Geometry: final body of the model. Coordinates: model frame, mm. Coordinates: 2 decimals unless noted, no trailing zeros. Write each loop counter-clockwise with the first axis right and the second up, starting at its lowest first coordinate (ties: lowest second). Pieces come first, ordered by that corner, then holes. Notation, with made-up numbers: (-22.75, 15) - (-13.75, 15) arc R9 cw to (-13.75, 22) - close; hole circle Ø2 at (36, 38). An arc over 180 degrees is marked (long way). Answer as a JSON object with one key per item and string values. Group by question number.
Item 1: Section A-A on y = 3.15. Return loops of the section in (x, z).
Item 2: First-contact query: pin 1 Ø2.5 at (x, y) = (-7.5, 3.5) entering from +Z; pin 2 Ø3 at (y, z) = (3.5, 14) entering from +X; pin 3 Ø1.5 at (y, z) = (3, -24.5) entering from +X. Flat tips, straight axial feed; report the tip coordinate or a pass-through.
Item 3: Section B-B on x = -16. Return loops of the section in (y, z), and give its area (4 significant figures).
Item 4: Line query: line 1 along Z through (x, y) = (5, 4.55); line 2 along X through (y, z) = (4.05, 21.5); line 3 along X through (y, z) = (3.55, 31). Output: solid intervals per line, ascending. Write a range as from..to.
Item 5: Section C-C on z = 12. Return loops of the section in (x, y), and give its area (3 significant figures).
```python
from build123d import *

# Parameters (mm, degrees)
BOSS_EXTRUDE1_DEPTH = 5


with BuildPart() as part:
    # Sketch1 → Boss-Extrude1 (new body)
    with BuildSketch(Plane(origin=(0, 0, 0), x_dir=(1, 0, 0), z_dir=(0, 1, 0))):
        with BuildLine():
            Line((48.939716241, 35.5), (-48.939716241, 35.5))
            ThreePointArc((-48.939716241, 35.5), (-52.484341475, 34.393332114), (-54.769665613, 31.46649501))
            Line((-54.769665613, 31.46649501), (-77.961623751, -30.089730331))
            ThreePointArc((-77.961623751, -30.089730331), (-77.507936909, -33.775842846), (-74.218478088, -35.5))
            Line((-74.218478088, -35.5), (-38.760968174, -35.5))
            ThreePointArc((-38.760968174, -35.5), (-35.349777153, -34.746684682), (-32.573080563, -32.626858226))
            Line((-32.573080563, -32.626858226), (-24.304233813, -22.837670888))
            ThreePointArc((-24.304233813, -22.837670888), (-21.561817428, -20.744015129), (-18.192739876, -20))
            Line((-18.192739876, -20), (0, -20))
            Line((0, -20), (18.192739876, -20))
            ThreePointArc((18.192739876, -20), (21.561817428, -20.744015129), (24.304233813, -22.837670888))
            Line((24.304233813, -22.837670888), (32.573080563, -32.626858226))
            ThreePointArc((32.573080563, -32.626858226), (35.349777153, -34.746684682), (38.760968174, -35.5))
            Line((38.760968174, -35.5), (74.218478088, -35.5))
            ThreePointArc((74.218478088, -35.5), (77.507936909, -33.775842846), (77.961623751, -30.089730331))
            Line((77.961623751, -30.089730331), (54.769665613, 31.46649501))
            ThreePointArc((54.769665613, 31.46649501), (52.484341475, 34.393332114), (48.939716241, 35.5))
        make_face()
    extrude(amount=BOSS_EXTRUDE1_DEPTH)


solid = part.part
```
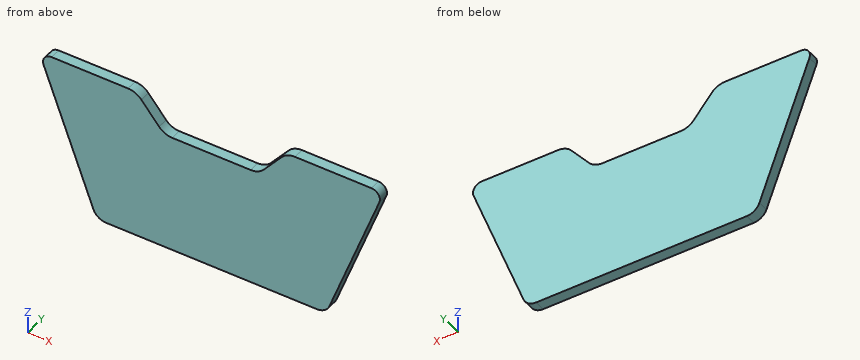
Checks:
{
 "1": {"outline": "(-77.96, 30.09) - (-54.77, -31.47) arc R6.23 ccw to (-48.94, -35.5) - (48.94, -35.5) arc R6.23 ccw to (54.77, -31.47) - (77.96, 30.09) arc R4 ccw to (74.22, 35.5) - (38.76, 35.5) arc R8.1 ccw to (32.57, 32.63) - (24.3, 22.84) arc R8 cw to (18.19, 20) - (-18.19, 20) arc R8 cw to (-24.3, 22.84) - (-32.57, 32.63) arc R8.1 ccw to (-38.76, 35.5) - (-74.22, 35.5) arc R4 ccw to start"},
 "2": {"pin 1": "z = 20", "pin 2": "x = 72.46", "pin 3": "x = 57.68"},
 "3": {"outline": "(0, -35.5) - (5, -35.5) - (5, 20) - (0, 20) - close", "area": "277.5 mm^2"},
 "4": {"line 1": "-35.5..20", "line 2": "-74.73..-22.86, 22.86..74.73", "line 3": "-78.19..-31.2, 31.2..78.19"},
 "5": {"outline": "(-71.15, 0) - (71.15, 0) - (71.15, 5) - (-71.15, 5) - close", "area": "711 mm^2"}
}
